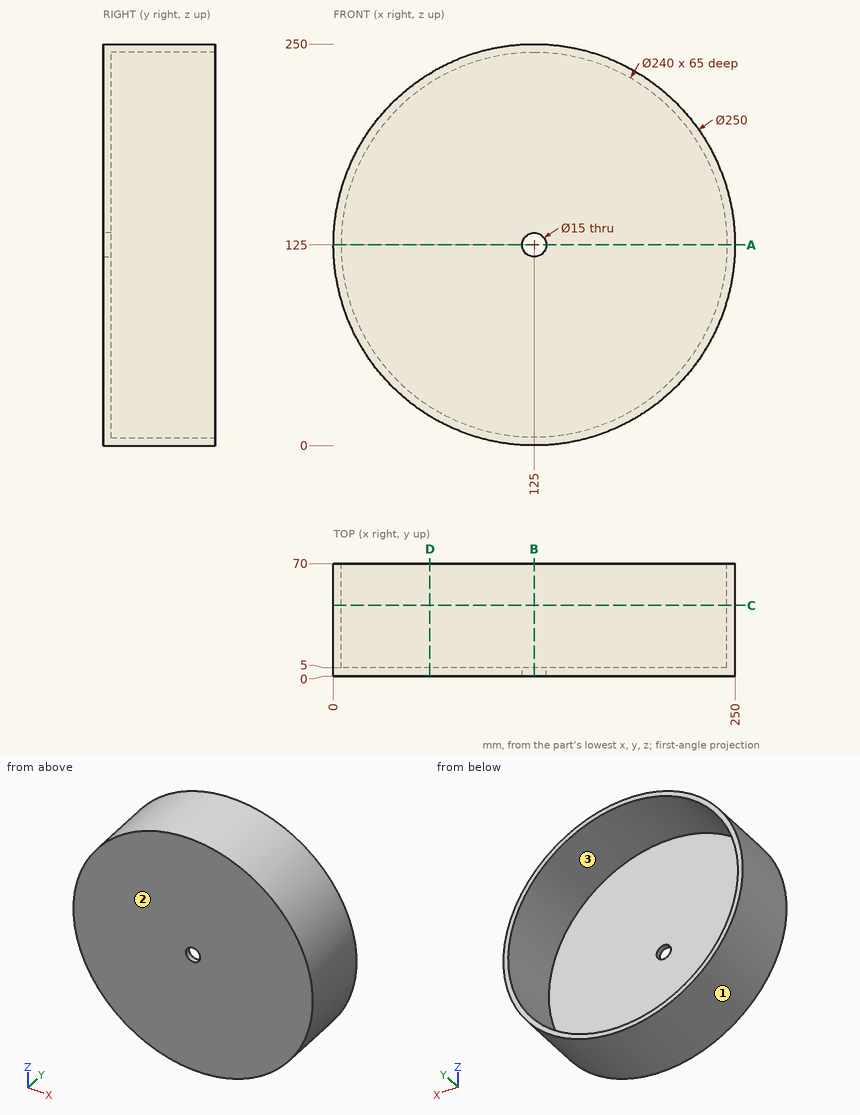
Here's the drawing with two shaded views (mm, measured from the low corner). I have some questions. Give positions to 0.01 mm unless a question says otherwise; leave off trailing zeros. Write each loop counter-clockwise with the first axis right and the second up, starting at its lowest first coordinate (ties: lowest second). Pieces come first, ordered by that corner, then holes. Notation, with made-up numbers: (6, 61.5) -> (23, 61.5) arc R28 ccw to (23, 79.5) -> close; hole circle Ø5 at (26, 86.25). An arc over 180 degrees is marked (long way). Answer as a JSON object with one key per item and string values. Group by question number.
Item 1: Suppose I cut it at A-A (z = 125). Please give me the cut outline in (x, y), plus the area to 4 significant figures.
Item 2: We'd pull the mould along Z, two halves only. Please class the marked faces 1, 2 and 3: +Z half, -Z half, draft (parallel to the pull), parting line (faces both ways), or undercut.
Item 3: I'm going to push flat-ended pins straight in: P1, Ø3, axis at y = 17.5, z = 32, coming from the -X side; P2, Ø3, axis at x = 57.5, z = 121, coming from the +Y side; P3, Ø6, axis at x = 221, y = 15, coming from the +Z side; P4, Ø13.5, axis at x = 125, z = 125, coming from the +Y side. Where does each tip first touch, or does it pass through?
Item 4: Suppose I cut it at C-C (y = 44). Please give me the cut outline in (x, z), plus the area to 3 significant figures.
Item 5: Suppose I cut it at B-B (x = 125). Please give me the cut outline in (y, z), plus the area to 4 significant figures.
Item 6: Suppose I cut it at D-D (x = 60). Please give me the cut outline in (y, z).
Item 7: Please list where these lines run through material, in increasing order: line 1 (X direction, y = 45.5, z = 125); line 2 (X direction, y = 1.45, z = 125); line 3 (Y direction, x = 92, z = 223). Write a range as [from, to].
Findings:
{
 "1": {"outline": "(0, 0) -> (117.5, 0) -> (117.5, 5) -> (5, 5) -> (5, 70) -> (0, 70) -> close; (132.5, 0) -> (250, 0) -> (250, 70) -> (245, 70) -> (245, 5) -> (132.5, 5) -> close", "area": "1,825 mm²"},
 "2": {"face 1": "parting line", "face 2": "draft", "face 3": "undercut"},
 "3": {"P1": "stops at x = 39.84", "P2": "stops at y = 5", "P3": "stops at z = 208.52", "P4": "passes through"},
 "4": {"outline": "circle Ø250 at (125, 125); hole circle Ø240 at (125, 125)", "area": "3,850 mm²"},
 "5": {"outline": "(0, 0) -> (70, 0) -> (70, 5) -> (5, 5) -> (5, 117.5) -> (0, 117.5) -> close; (0, 132.5) -> (5, 132.5) -> (5, 245) -> (70, 245) -> (70, 250) -> (0, 250) -> close", "area": "1,825 mm²"},
 "6": {"outline": "(0, 18.23) -> (70, 18.23) -> (70, 24.13) -> (5, 24.13) -> (5, 225.87) -> (70, 225.87) -> (70, 231.77) -> (0, 231.77) -> close"},
 "7": {"line 1": "x = [0, 5], [245, 250]", "line 2": "x = [0, 117.5], [132.5, 250]", "line 3": "y = [0, 5]"}
}
